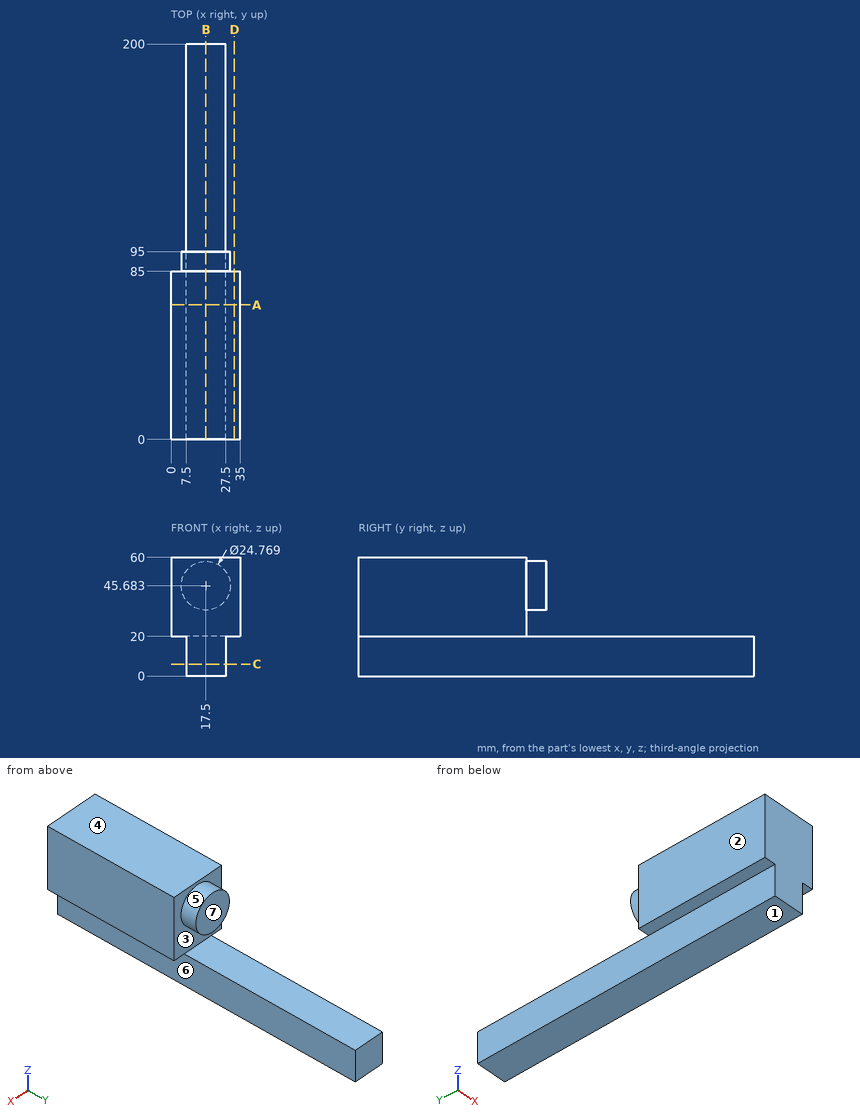
Design review of the part shown in the three views and the two pictorial views. Dimensions are in mm from the part's minimum x, y and z. A direction names the side the tool comes from. Give positions to 0.01 mm unless a question says otherwise; leave off trailing zeros. Write each loop counter-clockwise with the first axis right and the second up, starting at its lowest first coordinate (ties: lowest second). Pieces come first, ordered by that corner, then holes. Notation, with made-up numbers: M -17.5,88.5 L -11.5,88.5 A25 ccw -11.5,103.5 Z; hole C 57.5,13 d1. An arc over 180 degrees is marked long. Answer as CSV lines item,"result".
1. Consider section A-A, the plane y = 68. Write out the cut boundary in (x, z).
Findings:
outline,"M 0,20 L 7.5,20 L 7.5,0 L 27.5,0 L 27.5,20 L 35,20 L 35,60 L 0,60 Z"
2. For pin 1 (6 mm diameter, centred on y = 104, z = 7.5, fed in from +X); pin 2 (12 mm diameter, centred on x = 3.5, z = 52.5, fed in from +Y); pin 3 (6 mm diameter, centred on x = 14, y = 119, fed in from +Z); pin 4 (3 mm diameter, centred on x = 5.5, z = 12.5, fed in from +Y), all flat-tipped, find the tip position at first contact; note any pin that passes through.
Findings:
pin 1,"stops at x = 27.5"
pin 2,"stops at y = 95"
pin 3,"stops at z = 20"
pin 4,"passes through"
3. Consider section D-D, the plane x = 32. Write out the cut boundary in (y, z), then the cut area to 3 significant figures.
Findings:
outline,"M 0,20 L 85,20 L 85,60 L 0,60 Z"
area,"3,400 mm2"
4. For the marked faces 5, 6 and 7, list the 3-axis set-ups (+Z, -Z, +X, -X, +Y, -Y) from which the entire face can be reached by the end or side of a thin tool; tool diameter is ignored.
Findings:
face 5,"+Y"
face 6,"-Z, +X, +Y, -Y"
face 7,"+Z, +X, -X, +Y"
5. Draft analysis for pull direction Z (two halves, no side actions). For the marked faces 1, 2, 3 and 4, state which applies: +Z half, -Z half, draft (parallel to the pull), parting line (faces both ways), or undercut.
Findings:
face 1,"-Z half"
face 2,"draft"
face 3,"undercut"
face 4,"+Z half"
6. Consider section C-C, the plane z = 6. Write out the cut boundary in (x, y), then the cut area to 3 significant figures.
Findings:
outline,"M 7.5,0 L 27.5,0 L 27.5,200 L 7.5,200 Z"
area,"4,000 mm2"
7. Wall thickness on line 1 (Y direction, x = 11.5, z = 37.5); line 2 (Y direction, x = 20, z = 30); line 3 (Z direction, x = 12, y = 147.5): over which ranges is each line inside the solid? List them lowest first.
Findings:
line 1,"y = 0 to 95"
line 2,"y = 0 to 85"
line 3,"z = 0 to 20"
8. Consider section B-B, the plane x = 17.5. Write out the cut boundary in (y, z), then the cut area to 3 significant figures.
Findings:
outline,"M 0,0 L 200,0 L 200,20 L 85,20 L 85,33.3 L 95,33.3 L 95,58.07 L 85,58.07 L 85,60 L 0,60 Z"
area,"7,650 mm2"
